Read the model definition and answer for the solid it produces. Units are mm, in the model's axes. Face numbers are marked on the shaded views. A direction names the side the tool comes from. Give positions to 0.01 mm unless a question says otherwise; leave off trailing zeros. Loops run counter-clockwise (first coordinate to the right, second up) from the corner with the lowest first, then second, coordinate; pieces in that order, holes last. Notation, with made-up numbers: (28.5, 27.25) - (56.5, 27.25) arc R26 ccw to (56.5, 41.25) - close; hole circle Ø7 at (-8.75, -33.75). An arc over 180 degrees is marked (long way). Use a Markdown table: item, result. Add a question column.
Item 1: A cutting plane is placed at C-C (y = 116). Determine the outline of the cut face in (x, z).
Item 2: Consider probe 1 along X at (y, z) = (1, 0); probe 2 along X at (y, z) = (128.5, -57.5); probe 3 along Z at (x, y) = (-59.5, 82.5). Determine where each line is inside the solid, lowest interval first. Write a range as [from, to].
Item 3: A cutting plane is placed at A-A (x = -79.5). Determine the outline of the cut face in (y, z).
Item 4: Each of these flat-tipped pins is pushed along its axis until it touches: P1, Ø1, axis at x = -68, z = 19, coming from the +Y side; P2, Ø3, axis at x = -22.5, z = -78, coming from the +Y side; P3, Ø4.5, axis at y = 96.5, z = -78.5, coming from the -X side; P4, Ø4, axis at x = 15, z = 40, coming from the +Y side. Where does it stop, or does it pass through?
Item 5: A cutting plane is placed at B-B (z = 58). Determine the outline of the cut face in (x, y).
Item 6: For a pull along X with two mould halves and no side action, classify the marked faces 1, 2 and 3 as +X half, -X half, draft (parallel to the pull), parting line (faces both ways), or undercut.
Item 7: Which of the six approach directions +Z, -Z, +X, -X, +Y, -Y give full straight-line access (tool end or side, diameter ignored) to the marked faces 4 and 5?
from build123d import *

# Parameters (mm, degrees)
SKETCH1_W           = 215
SKETCH1_H           = 150
BOSS_EXTRUDE1_DEPTH = 4
SKETCH2_W           = 215
SKETCH2_H           = 150
SKETCH2_W_2         = 208
SKETCH2_H_2         = 142
BOSS_EXTRUDE2_DEPTH = 130
SKETCH4_W           = 180
SKETCH4_H           = 50
CUT_EXTRUDE1_DEPTH  = 6
FILLET1_R           = 5
FILLET2_R           = 5
FILLET3_R           = 5
FILLET4_R           = 5
SKETCH6_R           = 2.25
CUT_EXTRUDE2_DEPTH  = 6


with BuildPart() as part:
    # Sketch1 → Boss-Extrude1 (new body)
    with BuildSketch(Plane(origin=(0, 0, 0), x_dir=(1, 0, 0), z_dir=(0, 1, 0))):
        with Locations((0, 5)):
            Rectangle(SKETCH1_W, SKETCH1_H)
    extrude(amount=BOSS_EXTRUDE1_DEPTH)

    # Sketch2 → Boss-Extrude2 (add)
    with BuildSketch(Plane(origin=(0, 4, 0), x_dir=(1, 0, 0), z_dir=(0, 1, 0))):
        with Locations((0, 5)):
            Rectangle(SKETCH2_W, SKETCH2_H)
        with Locations((0, 5)):
            Rectangle(SKETCH2_W_2, SKETCH2_H_2, mode=Mode.SUBTRACT)
    extrude(amount=BOSS_EXTRUDE2_DEPTH)

    # Sketch4 → Cut-Extrude1 (cut)
    with BuildSketch(Plane(origin=(0, 0, -80), x_dir=(-1, 0, 0), z_dir=(0, 0, -1))):
        with Locations((0, 109)):
            Rectangle(SKETCH4_W, SKETCH4_H)
    extrude(amount=-CUT_EXTRUDE1_DEPTH, mode=Mode.SUBTRACT)

    # Fillet1
    fillet1_edges = [part.edges().sort_by_distance(p)[0] for p in [
        (-107.5, 67, -80),
    ]]
    fillet(fillet1_edges, radius=FILLET1_R)

    # Fillet2
    fillet2_edges = [part.edges().sort_by_distance(p)[0] for p in [
        (107.5, 67, -80),
    ]]
    fillet(fillet2_edges, radius=FILLET2_R)

    # Fillet3
    fillet3_edges = [part.edges().sort_by_distance(p)[0] for p in [
        (-107.5, 67, 70),
    ]]
    fillet(fillet3_edges, radius=FILLET3_R)

    # Fillet4
    fillet4_edges = [part.edges().sort_by_distance(p)[0] for p in [
        (107.5, 67, 70),
    ]]
    fillet(fillet4_edges, radius=FILLET4_R)

    # Sketch6 → Cut-Extrude2 (cut)
    with BuildSketch(Plane(origin=(0, 0, 0), x_dir=(-1, 0, 0), z_dir=(0, -1, 0))):
        with Locations(Location((15, -20, 0), (0, 0, 90))):
            Circle(SKETCH6_R)
        with Locations(Location((-15, -40, 0), (0, 0, 90))):
            Circle(SKETCH6_R)
        with Locations(Location((15, 0, 0), (0, 0, 90))):
            Circle(SKETCH6_R)
        with Locations(Location((-15, -20, 0), (0, 0, 90))):
            Circle(SKETCH6_R)
        with Locations(Location((15, 20, 0), (0, 0, 90))):
            Circle(SKETCH6_R)
        with Locations(Location((-15, 20, 0), (0, 0, 90))):
            Circle(SKETCH6_R)
        with Locations(Location((15, -40, 0), (0, 0, 90))):
            Circle(SKETCH6_R)
        with Locations(Location((-15, 0, 0), (0, 0, 90))):
            Circle(SKETCH6_R)
    extrude(amount=-CUT_EXTRUDE2_DEPTH, mode=Mode.SUBTRACT)


solid = part.part
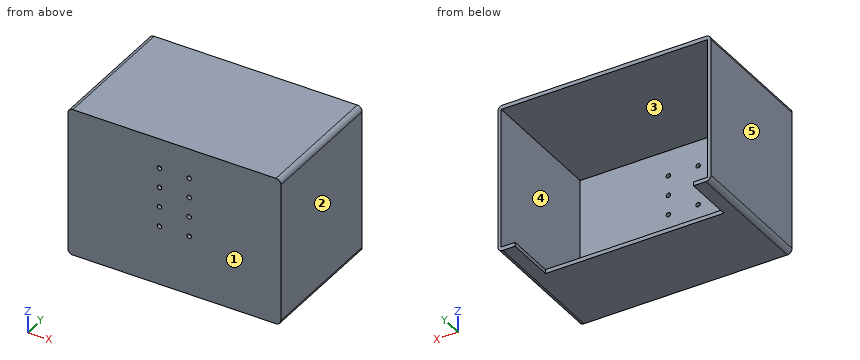
Geometry says:
| question | item | result |
|---|---|---|
| 1 | outline | (-107.5, -75) arc R5 ccw to (-102.5, -80) - (-90, -80) - (-90, -76) - (-104, -76) - (-104, 66) - (104, 66) - (104, -76) - (90, -76) - (90, -80) - (102.5, -80) arc R5 ccw to (107.5, -75) - (107.5, 65) arc R5 ccw to (102.5, 70) - (-102.5, 70) arc R5 ccw to (-107.5, 65) - close |
| 2 | probe 1 | [-107.5, -17.25], [-12.75, 12.75], [17.25, 107.5] |
| 2 | probe 2 | [-107.5, -104], [104, 107.5] |
| 2 | probe 3 | [-80, -76], [66, 70] |
| 3 | outline | (0, -80) - (84, -80) - (84, -76) - (4, -76) - (4, 66) - (134, 66) - (134, 70) - (0, 70) - close |
| 4 | P1 | y = 4 |
| 4 | P2 | y = 84 |
| 4 | P3 | x = -107.34 |
| 4 | P4 | through |
| 5 | outline | (-107.5, 0) - (107.5, 0) - (107.5, 134) - (104, 134) - (104, 4) - (-104, 4) - (-104, 134) - (-107.5, 134) - close |
| 6 | face 1 | draft |
| 6 | face 2 | +X half |
| 6 | face 3 | undercut |
| 7 | face 4 | +Y |
| 7 | face 5 | +Z, -Z, -X, +Y, -Y |
